```python
from build123d import *

# Parameters (mm, degrees)
F1_DEPTH = 25
F2_R     = 5.5
F2_R_2   = 4.5
F3_DEPTH = 5
F4_DEPTH = 5
F6_DEPTH = 5


# Not quite as in the source:
# - ends of sketch curves that miss each other by under 0.0002 mm in the source are joined


with BuildPart() as f1:
    # F0 (on Front) → F1 (new body)
    with BuildSketch(Plane.XZ):
        with BuildLine():
            Line((134, 0), (134, 5))
            Line((134, 5), (5, 5))
            ThreePointArc((5, 5), (2.4118095455, 4.6592580848), (0, 3.6602538402))
            Line((0, 3.6602538402), (0, 0))
            Line((0, 0), (5, 0))
            Line((5, 0), (134, 0))
        make_face()
        with BuildLine():
            Line((0, 0), (0, 3.6602538402))
            ThreePointArc((0, 3.6602538402), (-3.6602539143, -1.284e-07), (-4.9999998289, -5))
            Line((-4.9999998289, -5), (-5, -56))
            Line((-5, -56), (0, -56))
            Line((0, -56), (0, -5))
            Line((0, -5), (0, 0))
        make_face()
        with BuildLine():
            ThreePointArc((0, -5), (1.4644660941, -1.4644660941), (5, 0))
            Line((5, 0), (0, 0))
            Line((0, 0), (0, -5))
        make_face()
    extrude(amount=-F1_DEPTH)

    # F2 (on face) → F3 (cut)
    with BuildSketch(Plane.XY.offset(5)):
        with Locations((114, 12.5)):
            Circle(F2_R)
        with Locations((84, 12.5)):
            Circle(F2_R_2)
        with Locations((45, 12.5)):
            Circle(F2_R_2)
    extrude(amount=-F3_DEPTH, mode=Mode.SUBTRACT)

    # F2 (on face) → F4 (cut)
    with BuildSketch(Plane.XY.offset(5)):
        with Locations((114, 12.5)):
            Circle(F2_R)
        with Locations((84, 12.5)):
            Circle(F2_R_2)
        with Locations((45, 12.5)):
            Circle(F2_R_2)
    extrude(amount=-F4_DEPTH, mode=Mode.SUBTRACT)

    # F5 (on face) → F6 (cut)
    with BuildSketch(Plane(origin=(-5, 0, 0), x_dir=(0, -1, 0), z_dir=(-1, 0, 0))):
        with BuildLine():
            ThreePointArc((-12.5, -50.5), (-9.3180194847, -49.1819805153), (-8, -46))
            ThreePointArc((-8, -46), (-15.6819805153, -42.8180194847), (-12.5, -50.5))
        make_face()
    extrude(amount=-F6_DEPTH, mode=Mode.SUBTRACT)


solid = f1.part
```
For this review, take the finished solid that the model builds, in its own axes (mm). A direction names the side the tool comes from. Give positions to 0.01 mm unless a question says otherwise; leave off trailing zeros. Loops run counter-clockwise (first coordinate to the right, second up) from the corner with the lowest first, then second, coordinate; pieces in that order, holes last. Notation, with made-up numbers: M 76.5,39 L 114.5,39 A26 cw 114.5,64 Z; hole C -31,-10.5 d8. An arc over 180 degrees is marked long. One line per item, written item: value. Start each with the question number.
Q1. Add section D-D (y = 4). Give the boundary of the cut face in (x, z).
Q2. Clearance check with flat-ended pins moving along their axes: pin 1 Ø12 at (y, z) = (7.5, -29.5) entering from +X; pin 2 Ø5 at (x, y) = (108.5, 20.5) entering from -Z. State where each tip first meets the part, or that it passes through.
Q3. Add section B-B (y = 14.5). Give the boundary of the cut face in (x, z).
Q4. Add section A-A (x = 45). Give the boundary of the cut face in (y, z), and give its area (3 significant figures).
Q5. For L1, parallel to Y at x = 84, z = 1; L2, parallel to Y at x = 114, z = 2; L3, parallel to Z at x = 37.5, y = 17, list the stretches that pass through material, from the lowest coordinate up.
Q6. Draft analysis for pull direction Y (two halves, no side actions). For faces 1 (the face through (1, 12, -2)), 2 (the face through (79.504, 12.698, 2.535)), 3 (the face through (44, 0, 2)), state which applies: released by +Y, released by -Y, zero draft, split by the parting line, or undercut.
Q7. Add section C-C (z = -49). Give the boundary of the cut face in (x, y), and give its area (3 significant figures).
Q8. Machinability: for faces 4 (the face through (-5, 12, -30)), 5 (the face through (69, 12, 0)), which of the approach directions +Z, -Z, +X, -X, +Y, -Y give a long, thin tool a straight path to every point of the face, cutting with its end or side? Answer none if there is none.
Reply:
1. outline: M -5,-56 L 0,-56 L 0,-5 A5 cw 5,0 L 134,0 L 134,5 L 5,5 A10 ccw 0,3.66 A10 ccw -5,-5 Z
2. pin 1: x = 0
2. pin 2: z = 0
3. outline: M -5,-56 L 0,-56 L 0,-50.03 L -5,-50.03 Z; M -5,-41.97 L 0,-41.97 L 0,-5 A5 cw 5,0 L 40.97,0 L 40.97,5 L 5,5 A10 ccw 0,3.66 A10 ccw -5,-5 Z; M 49.03,0 L 79.97,0 L 79.97,5 L 49.03,5 Z; M 88.03,0 L 108.88,0 L 108.88,5 L 88.03,5 Z; M 119.12,0 L 134,0 L 134,5 L 119.12,5 Z
4. outline: M 0,0 L 8,0 L 8,5 L 0,5 Z; M 17,0 L 25,0 L 25,5 L 17,5 Z
4. area: 80.0 mm²
5. L1: 0 to 8, 17 to 25
5. L2: 0 to 7, 18 to 25
5. L3: 0 to 5
6. face 1: zero draft
6. face 2: undercut
6. face 3: released by -Y
7. outline: M -5,0 L 0,0 L 0,9.15 L -5,9.15 Z; M -5,15.85 L 0,15.85 L 0,25 L -5,25 Z
7. area: 91.5 mm²
8. face 4: +Z, -Z, -X, +Y, -Y
8. face 5: -Z, +X, +Y, -Y
